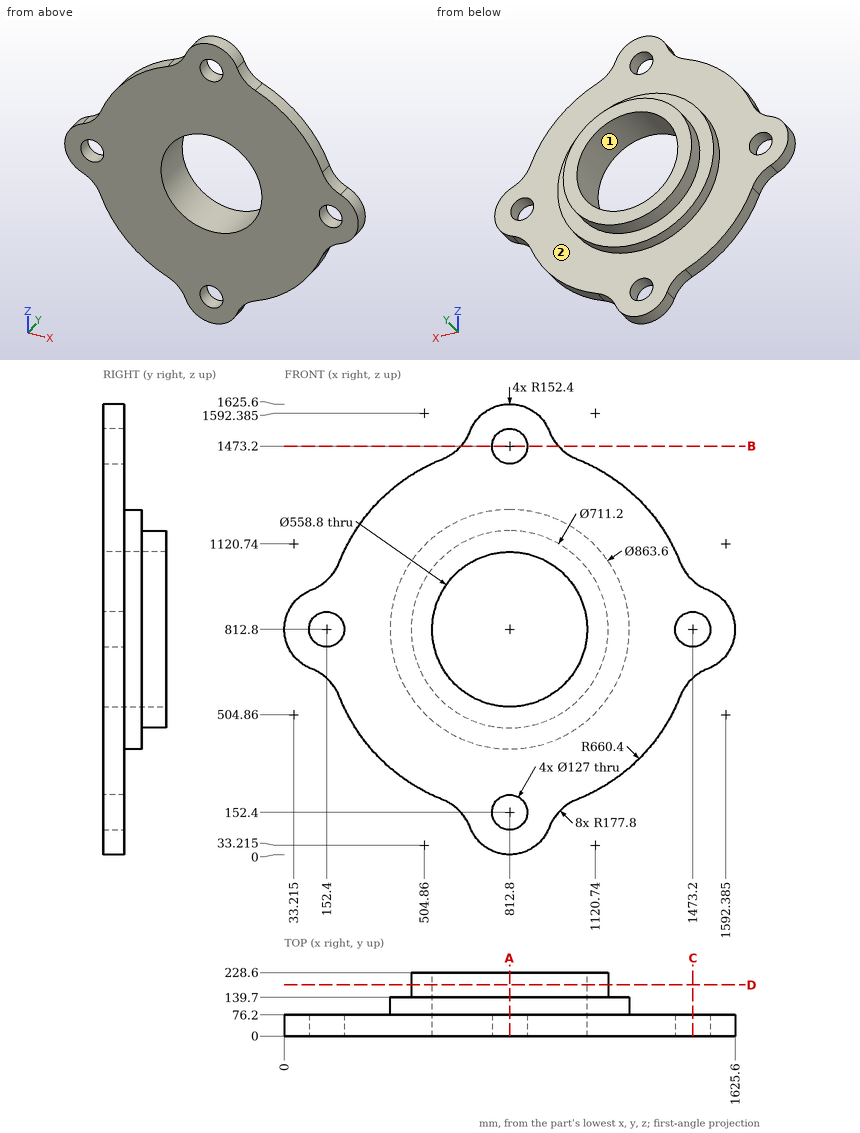
Input: dimensioned drawing with shaded views. Units: mm. Origin: part minimum x, y, z. A direction names the side the tool comes from. Coordinates: 2 decimals unless noted, no trailing zeros. Write each loop counter-clockwise with the first axis right and the second up, starting at its lowest first coordinate (ties: lowest second). Pieces come first, ordered by that corner, then holes. Notation, with made-up numbers: M 59.5,4 L 116.5,4 A7 cw 116.5,13 Z; hole C 14.5,-4.75 d8. An arc over 180 degrees is marked long. Answer as CSV lines item,"result". Start each with the question number.
Q1. Cut plane B-B on z = 1473.2. Return the cut outline in (x, y).
Q2. Line query: line 1 (X direction, y = 51, z = 812.8); line 2 (Y direction, x = 996, z = 342). Output: solid intervals per line, ascending. Write a range as from..to.
Q3. Reachability of the marked faces 1 and 2 from +Z, -Z, +X, -X, +Y, -Y: full face, straight path, thin tool, end or side. Return the list, or none.
Q4. Cut plane A-A on x = 812.8. Return the cut outline in (y, z), then the cut area to 3 significant figures.
Q5. Cut plane C-C on x = 1473.2. Return the cut outline in (y, z), then the cut area to 3 significant figures.
Q6. Pin query (flat end, axial travel): P1, Ø12, axis at x = 787, y = 155.5, coming from the -Z side; P2, Ø3, axis at x = 711.5, z = 1198.5, coming from the +Y side; P3, Ø10, axis at y = 200.5, z = 1066, coming from the +X side; P4, Ø1, axis at x = 819, z = 1193.5, coming from the -Y side. Return the tip coordinate at first contact, or that it passes through.
Q7. Cut plane D-D on y = 184. Return the cut outline in (x, z).
Findings below:
1,outline,"M 636.8,0 L 749.3,0 L 749.3,76.2 L 636.8,76.2 Z; M 876.3,0 L 988.8,0 L 988.8,76.2 L 876.3,76.2 Z"
2,line 1,"x = 0..88.9, 215.9..533.4, 1092.2..1409.7, 1536.7..1625.6"
2,line 2,"y = 0..76.2"
3,face 1,"+Y, -Y"
3,face 2,"+Y"
4,outline,"M 0,0 L 76.2,0 L 76.2,88.9 L 0,88.9 Z; M 0,215.9 L 76.2,215.9 L 76.2,381 L 139.7,381 L 139.7,457.2 L 228.6,457.2 L 228.6,533.4 L 0,533.4 Z; M 0,1092.2 L 228.6,1092.2 L 228.6,1168.4 L 139.7,1168.4 L 139.7,1244.6 L 76.2,1244.6 L 76.2,1409.7 L 0,1409.7 Z; M 0,1536.7 L 76.2,1536.7 L 76.2,1625.6 L 0,1625.6 Z"
4,area,"94,800 mm2"
5,outline,"M 0,636.8 L 76.2,636.8 L 76.2,749.3 L 0,749.3 Z; M 0,876.3 L 76.2,876.3 L 76.2,988.8 L 0,988.8 Z"
5,area,"17,100 mm2"
6,P1,"stops at z = 457.75"
6,P2,"stops at y = 139.7"
6,P3,"stops at x = 1067.45"
6,P4,"stops at y = 0"
7,outline,"C 812.8,812.8 d711.2; hole C 812.8,812.8 d558.8"
